Could you check a few things on this model? Use its own coordinates, in mm. Give positions to 0.01 mm unless a question says otherwise; leave off trailing zeros. Order: outer loops, then holes, each group sorted by start corner. A loop starts at its lowest first (then second) coordinate and runs counter-clockwise, first axis right, second up.
(1) Imagine slicing it at C-C, the plane x = 3.75. Write out the boundary of the cut face in (y, z), then the cut area to 3 significant figures.
(2) Will this pin go through, and if not, where does the flat tip stop? pin 1 (8 mm diameter, centred on y = -15, z = 21, fed in from +X).
(3) Imagine slicing it at A-A, the plane y = 0. Write out the boundary of the cut face in (x, z).
(4) If I drill on probe 1 along Y at (x, z) = (1.5, -39); probe 2 along Y at (x, z) = (3, 26.5); probe 3 along Y at (x, z) = (4.75, 3), over which ranges is the centre line in solid material (lowest first)?
from build123d import *

# Parameters (mm, degrees)
ESQUISSE1_R             = 45
ESQUISSE1_R_2           = 32
BOSS_EXTRU_1_DEPTH      = 7
ESQUISSE3_R             = 2.5
ESQUISSE3_R_2           = 4
ENL_V_MAT_EXTRU_1_DEPTH = 65.02343321
BOSS_EXTRU_3_START      = -7
ESQUISSE4_W             = 90
ESQUISSE4_H             = 90
ESQUISSE4_R             = 32
BOSS_EXTRU_3_DEPTH      = 7
ESQUISSE5_R             = 2
ENL_V_MAT_EXTRU_2_DEPTH = 65.02343321
CONG_1_R                = 5


with BuildPart() as part:
    # Esquisse1 → Boss.-Extru.1 (new body)
    with BuildSketch(Plane(origin=(0, 0, 0), x_dir=(0, 0, -1), z_dir=(1, 0, 0))):
        Circle(ESQUISSE1_R)
        Circle(ESQUISSE1_R_2, mode=Mode.SUBTRACT)
    extrude(amount=BOSS_EXTRU_1_DEPTH)

    # Esquisse3 → Enlèv. mat.-Extru.1 (cut, through all)
    with BuildSketch(Plane(origin=(7, 0, 0), x_dir=(0, 0, -1), z_dir=(1, 0, 0))):
        with Locations((0, 38)):
            Circle(ESQUISSE3_R)
        with Locations((32.908965344, 19)):
            Circle(ESQUISSE3_R)
        with Locations((32.908965344, -19)):
            Circle(ESQUISSE3_R)
        with Locations((0, -38)):
            Circle(ESQUISSE3_R)
        with Locations((-32.908965344, -19)):
            Circle(ESQUISSE3_R)
        with Locations((-32.908965344, 19)):
            Circle(ESQUISSE3_R)
        with Locations((-20.848699038, 32.366367551)):
            Circle(ESQUISSE3_R_2)
        with Locations((38.454446046, 1.872319227)):
            Circle(ESQUISSE3_R_2)
        with Locations((-17.605747008, -34.238686778)):
            Circle(ESQUISSE3_R_2)
    extrude(amount=-ENL_V_MAT_EXTRU_1_DEPTH, mode=Mode.SUBTRACT)

    # Esquisse4 → Boss.-Extru.3 (add)
    with BuildSketch(Plane(origin=(7, 0, 0), x_dir=(0, 0, -1), z_dir=(1, 0, 0)).offset(BOSS_EXTRU_3_START)):
        Rectangle(ESQUISSE4_W, ESQUISSE4_H)
        Circle(ESQUISSE4_R, mode=Mode.SUBTRACT)
    extrude(amount=BOSS_EXTRU_3_DEPTH)

    # Esquisse5 → Enlèv. mat.-Extru.2 (cut, through all)
    with BuildSketch(Plane.ZY):
        with Locations((-39, 39)):
            Circle(ESQUISSE5_R)
        with Locations(Location((39, 39, 0), (0, 0, 180))):
            Circle(ESQUISSE5_R)
        with Locations((39, -39)):
            Circle(ESQUISSE5_R)
        with Locations(Location((-39, -39, 0), (0, 0, 180))):
            Circle(ESQUISSE5_R)
    extrude(amount=-ENL_V_MAT_EXTRU_2_DEPTH, mode=Mode.SUBTRACT)

    # Congé1
    cong_1_edges = [part.edges().sort_by_distance(p)[0] for p in [
        (3.5, -45, 45),
        (3.5, 45, 45),
        (3.5, -45, -45),
        (3.5, 45, -45),
    ]]
    fillet(cong_1_edges, radius=CONG_1_R)


solid = part.part
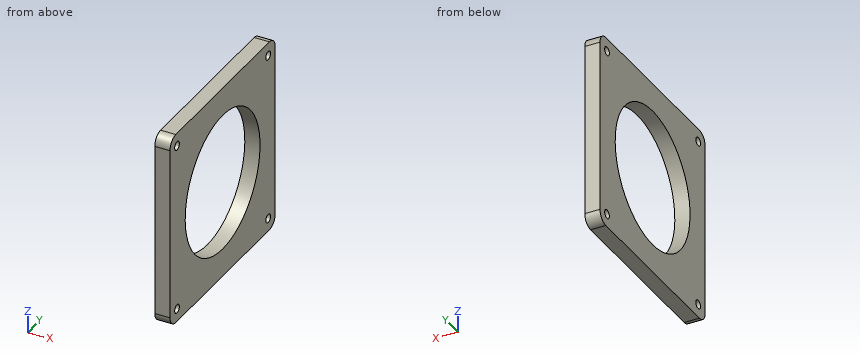
Answer block:
1. outline: (-45, -40) arc R5 ccw to (-40, -45) - (40, -45) arc R5 ccw to (45, -40) - (45, 40) arc R5 ccw to (40, 45) - (-40, 45) arc R5 ccw to (-45, 40) - close; hole circle Ø4 at (-39, -39); hole circle Ø4 at (-39, 39); hole circle Ø64 at (0, 0); hole circle Ø4 at (39, -39); hole circle Ø4 at (39, 39)
1. area: 4,810 mm2
2. pin 1: passes through
3. outline: (0, -45) - (7, -45) - (7, -32) - (0, -32) - close; (0, 32) - (7, 32) - (7, 45) - (0, 45) - close
4. probe 1: y = -45 to -41, -37 to 37, 41 to 45
4. probe 2: y = -45 to -17.94, 17.94 to 45
4. probe 3: y = -45 to -31.86, 31.86 to 45
